```python
from build123d import *

# Parameters (mm, degrees)
HEX_START     = -1.896533
HEX_2_DEPTH   = 1.896533
CHAMFER1_SIZE = 0.127
FILLET1_R     = 0.0635


with BuildPart() as part:
    # Sketch1 → Body (revolve)
    with BuildSketch(Plane(origin=(0, 0, 0), x_dir=(1, 0, 0), z_dir=(0, 1, 0))):
        Polygon((0, 0), (0, 2.3241), (2.8448, 2.3241), (2.8448, 1.4224), (15.5448, 1.4224), (15.5448, 0), align=None)
    revolve(axis=Axis((15.5448, 0, 0), (-1, 0, 0)))

    # Sketch2 → Hex 2 (cut)
    with BuildSketch(Plane.ZY.offset(HEX_START)):
        Polygon((-1.374815329, 0), (-0.687407664, -1.190625), (0.687407664, -1.190625), (1.374815329, 0), (0.687407664, 1.190625), (-0.687407664, 1.190625), align=None)
    extrude(amount=HEX_2_DEPTH, mode=Mode.SUBTRACT)

    # Chamfer1
    chamfer1_edges = [part.edges().sort_by_distance(p)[0] for p in [
        (0, 0, 2.3241),
        (15.5448, 0, 1.4224),
    ]]
    chamfer(chamfer1_edges, length=CHAMFER1_SIZE)

    # Fillet1
    fillet1_edges = [part.edges().sort_by_distance(p)[0] for p in [
        (2.8448, 0, 1.4224),
    ]]
    fillet(fillet1_edges, radius=FILLET1_R)

    # Hex Chamfer cone 1 section (through the dimple's axis) → Hex Chamfer (revolve, cut)
    with BuildSketch(Plane.ZX):
        Polygon((0, 0), (1.374815329, 0), (0, 1.374815329), align=None)
    revolve(axis=Axis((0, 0, 0), (1, 0, 0)), mode=Mode.SUBTRACT)


solid = part.part
```
Read the model definition and answer for the solid it produces. Units are mm, in the model's axes. A direction names the side the tool comes from. Give positions to 0.01 mm unless a question says otherwise; leave off trailing zeros. Write each loop counter-clockwise with the first axis right and the second up, starting at its lowest first coordinate (ties: lowest second). Pieces come first, ordered by that corner, then holes. Notation, with made-up numbers: (51.25, 79) -> (82.25, 79) arc R21 ccw to (82.25, 117) -> close; hole circle Ø4 at (18, 17). An arc over 180 degrees is marked (long way). Answer in a Markdown table with one row per item.
1) A tool of negligible diameter and unlimited length cuts with its end or side. For faces 5 (the flat face through (2.845, 2, 0)), 6 (the flat face through (0.962, -0.587, -1.036)), 7 (the cylindrical face through (1.5, 2.27, 0.5)), from which of +Z, -Z, +X, -X, +Y, -Y can it reach the whole face along a straight path? Write none if from no direction.
Results list:
| item | result |
|---|---|
| face 5 | +X |
| face 6 | -X |
| face 7 | +X, -X |
2) Determine the mould class of faces 1 (the flat face through (1, -1.191, 0)), 2 (the flat face through (15.545, 0, 0)), 3 (the cylindrical face through (9.25, 1.39, 0.31)), 4 (the flat face through (0.96, 0.6, -1.03)) for opening direction Z: released by +Z, released by -Z, zero draft, split by the parting line, or undercut.
Results list:
| item | result |
|---|---|
| face 1 | undercut |
| face 2 | zero draft |
| face 3 | split by the parting line |
| face 4 | undercut |
3) Section B-B on z = 0 is taken. Give the vertices of the cut face in (x, y).
Results list:
| item | result |
|---|---|
| outline | (0, -2.2) -> (0.13, -2.32) -> (2.84, -2.32) -> (2.84, -1.49) arc R0.06 cw to (2.91, -1.42) -> (15.42, -1.42) -> (15.54, -1.3) -> (15.54, 1.3) -> (15.42, 1.42) -> (2.91, 1.42) arc R0.06 cw to (2.84, 1.49) -> (2.84, 2.32) -> (0.13, 2.32) -> (0, 2.2) -> (0, 1.37) -> (0.18, 1.19) -> (1.9, 1.19) -> (1.9, -1.19) -> (0.18, -1.19) -> (0, -1.37) -> close |
4) Section A-A on x = 1.5 is taken. Give the vertices of the cut face in (y, z).
Results list:
| item | result |
|---|---|
| outline | circle Ø4.65 at (0, 0); hole (-1.19, -0.69) -> (0, -1.37) -> (1.19, -0.69) -> (1.19, 0.69) -> (0, 1.37) -> (-1.19, 0.69) -> close |
5) Section C-C on x = 9.75 is taken. Give the vertices of the cut face in (y, z), plus the area to 3 significant figures.
Results list:
| item | result |
|---|---|
| outline | circle Ø2.84 at (0, 0) |
| area | 6.36 mm^2 |
6) Straight lines are drawn through the part: line 1 (X direction, y = 1.4, z = -1.1); line 2 (X direction, y = -0.9, z = 0.25); line 3 (Z direction, x = 7.5, y = 0.05). For each, find the intervals that lie inside material, in ascending order. Write a range as [from, to].
Results list:
| item | result |
|---|---|
| line 1 | [0, 2.84] |
| line 2 | [1.9, 15.54] |
| line 3 | [-1.42, 1.42] |
7) Each of these flat-tipped pins is pushed along its axis until it touches: pin 1 Ø1.5 at (y, z) = (-1, 1) entering from -X; pin 2 Ø0.7 at (y, z) = (-0.5, 0.5) entering from -X; pin 3 Ø1.5 at (x, z) = (12.5, -1.5) entering from +Y. Where does it stop, or does it pass through?
Results list:
| item | result |
|---|---|
| pin 1 | x = 0 |
| pin 2 | x = 1.9 |
| pin 3 | y = 1.21 |
